```python
from build123d import *

# Parameters (mm, degrees)
EXTRUDE_START               = -0.5
EXTRUDE_1_OUTLINE_R         = 6.035
EXTRUDE_1_DEPTH             = 4.5
EXTRUDE_START_2             = 4
EXTRUDE_1_2_DEPTH           = 1
SKETCH_2_R                  = 6.035
EXTRUDE_2_DEPTH             = 4
CUT_EXTRUDE_1_DEPTH         = 2
CUT_EXTRUDE_2_DEPTH         = 5.5
HOLE_WIZARD_3_4_3_4_1_D     = 3.4
HOLE_WIZARD_3_4_3_4_1_DEPTH = 13
CHAMFER_1_SIZE              = 0.5


with BuildPart() as part:
    # 凸台-拉伸1: read off the stored shape, not the designer's step
    # 凸台-拉伸1 outline → 凸台-拉伸1 (new body)
    with BuildSketch(Plane.XY.offset(5).offset(EXTRUDE_START)):
        with Locations((-1.25, 0)):
            Circle(EXTRUDE_1_OUTLINE_R)
    extrude(amount=EXTRUDE_1_DEPTH)

    # Extrude 1 2 outline → Extrude 1 2 (add)
    with BuildSketch(Plane.XY.offset(EXTRUDE_START_2)):
        with BuildLine():
            ThreePointArc((0, -7.141428429), (8.5, 0), (0, 7.141428429))
            ThreePointArc((0, 7.141428429), (-8.5, 0), (0, -7.141428429))
        make_face()
    extrude(amount=EXTRUDE_1_2_DEPTH)

    # Extrude 1 3 outline → Extrude 1 3 (revolve, cut)
    with BuildSketch(Plane(origin=(-1.25, 0, 0), x_dir=(1, 0, 0), z_dir=(0, -1, 0))):
        Polygon((7.25, 5), (7.75, 4.5), (9.75, 4.5), (9.75, 5), align=None)
    revolve(axis=Axis((-1.25, 0, 0), (0, 0, 1)), mode=Mode.SUBTRACT)

    # Extrude 1 4 outline → Extrude 1 4 (revolve, cut)
    with BuildSketch(Plane(origin=(1.25, 0, 0), x_dir=(1, 0, 0), z_dir=(0, -1, 0))):
        Polygon((9.75, 4.5), (7.75, 4.5), (7.25, 4), (9.75, 4), align=None)
    revolve(axis=Axis((1.25, 0, 0), (0, 0, 1)), mode=Mode.SUBTRACT)

    # 草图2 → 凸台-拉伸2 (add)
    with BuildSketch(Plane(origin=(0, 0, 4), x_dir=(-1, 0, 0), z_dir=(0, 0, -1))):
        with Locations(Location((-1.25, 0, 0), (0, 0, 180))):
            Circle(SKETCH_2_R)
    extrude(amount=EXTRUDE_2_DEPTH)

    # 草图3 → 切除-拉伸1 (cut)
    with BuildSketch(Plane(origin=(0, 0, 0), x_dir=(-1, 0, 0), z_dir=(0, 0, -1))):
        Polygon((-6, -1.732050808), (-3.16, -1.732050808), (0, -3.556477658), (3.08, -1.778238829), (3.08, 1.778238829), (0, 3.556477658), (-3.16, 1.732050808), (-6, 1.732050808), align=None)
    extrude(amount=-CUT_EXTRUDE_1_DEPTH, mode=Mode.SUBTRACT)

    # 草图4 → 切除-拉伸2 (cut)
    with BuildSketch(Plane(origin=(0, 0, 2), x_dir=(-1, 0, 0), z_dir=(0, 0, -1))):
        Polygon((-3.08, -1.778238829), (0, -3.556477658), (3.08, -1.778238829), (3.08, 1.778238829), (0, 3.556477658), (-3.08, 1.778238829), align=None)
    extrude(amount=-CUT_EXTRUDE_2_DEPTH, mode=Mode.SUBTRACT)

    # 草图5 → 旋转1 (revolve)
    with BuildSketch(Plane.XZ, mode=Mode.PRIVATE) as revolve_1_sk:
        Polygon((3.05, 13), (0, 13), (0, 9), (3.75, 9), (3.75, 10), (3.05, 10), align=None)
    revolve(revolve_1_sk.sketch.rotate(Axis((0, 0, 13), (0, 0, -1)), 180), axis=Axis((0, 0, 13), (0, 0, -1)))

    # Ø3.4 (3.4) 直径孔1
    with Locations(Plane.XY.offset(13)):
        with Locations((0, 0)):
            Hole(HOLE_WIZARD_3_4_3_4_1_D / 2, depth=HOLE_WIZARD_3_4_3_4_1_DEPTH)

    # 倒角1
    chamfer_1_edges = [part.edges().sort_by_distance(p)[0] for p in [
        (4.58, -1.732050808, 0),
        (4.58, 1.732050808, 0),
    ]]
    chamfer(chamfer_1_edges, length=CHAMFER_1_SIZE)


solid = part.part
```
Verification items for the finished model (mm, model axes). A direction names the side the tool comes from. Round coordinates to 2 decimals unless told otherwise and drop trailing zeros.
1. Gauge pin test, flat ends, axial feed: P1, Ø7.5, axis at x = 6.5, y = 0, coming from the +Z side; P2, Ø6, axis at y = -3.5, z = 5.5, coming from the +X side; P3, Ø1.1, axis at y = -0.5, z = 6, coming from the -X side (3 decimals); P4, Ø1.8, axis at x = -1, y = 0.5, coming from the -Z side. Record the tip position at first contact, or that the pin passes through.
2. Access from +Z, -Z, +X, -X, +Y, -Y to the whole of each face (thin tool, end or side, straight path). Record for faces 5 (the flat face through (3, 3, 0)), 6 (the cylindrical face through (0.464, -5.984, 2.028)), 7 (the cylindrical face through (4.506, 1.813, 6.972)).
3. Draft check along X on faces 1 (the cylindrical face through (-2.02, 3.16, 9.51)), 2 (the flat face through (6, 0, 1)), 3 (the flat face through (7, 1, 4.5)), 4 (the conical face through (-6.134, 0.144, 4.135)). Enter one of: +X half, -X half, draft (parallel to the pull), parting line (faces both ways), or undercut.
4. Scan lines: L1, parallel to Y at x = 0, z = 9.15; L2, parallel to Y at x = 0, z = 11.75; L3, parallel to Z at x = -2.75, y = 3.75. Record each from-to range of solid material in increasing order.
Answer:
1. P1: stops at z = 13
1. P2: stops at x = 8.47
1. P3: stops at x = -7.285
1. P4: stops at z = 7.5
2. face 5: -Z, +X, -X, +Y, -Y
2. face 6: -Z
2. face 7: +Z
3. face 1: parting line
3. face 2: undercut
3. face 3: draft
3. face 4: -X half
4. L1: y = -3.75 to -1.7, 1.7 to 3.75
4. L2: y = -3.05 to -1.7, 1.7 to 3.05
4. L3: z = 0 to 9
